Can you work these out from the model? Positions are in its coordinate system, mm. Face numbers are marked on the shaded views. Give positions to 0.01 mm unless a question says otherwise; leave off trailing zeros. Order: outer loops, then holes, each group sorted by start corner. A loop starts at its lowest first (then second) coordinate and runs counter-clockwise, first axis right, second up. Notation, with made-up numbers: (5, 76) - (29, 76) arc R23 cw to (29, 108) - close; hole circle Ø7 at (25.5, 36). An arc over 180 degrees is marked (long way). One line per question, with ' | ' between items.
```python
from build123d import *

# Parameters (mm, degrees)
F0_R        = 2.5
F1_DEPTH    = 5
F2_R        = 0.1
F3_T1_DEPTH = 5.0886751346


# Not quite as in the source:
# - a fillet or chamfer that OpenCascade refuses, or shapes differently, is made with other operations: its cross-section is extruded or revolved along the edge and cut away or added


with BuildPart() as f1:
    # F0 (on Top) → F1 (new body)
    with BuildSketch(Plane.XY):
        Polygon((2.8867513459, 5), (-2.8867513459, 5), (-5.7735026919, 0), (-2.8867513459, -5), (2.8867513459, -5), (5.7735026919, 0), align=None)
        Circle(F0_R, mode=Mode.SUBTRACT)
    extrude(amount=F1_DEPTH)

    # F2
    f2_edges = [f1.edges().sort_by_distance(p)[0] for p in [
        (4.330127, 2.5, 0),
        (0, 5, 0),
        (-4.330127, 2.5, 0),
        (-4.330127, -2.5, 0),
        (0, -5, 0),
        (4.330127, -2.5, 0),
        (-2.5, 0, 0),
        (4.330127, 2.5, 5),
        (0, 5, 5),
        (-4.330127, 2.5, 5),
        (-4.330127, -2.5, 5),
        (0, -5, 5),
        (4.330127, -2.5, 5),
        (-2.5, 0, 5),
    ]]
    fillet(f2_edges, radius=F2_R)

    # F3: fillet of radius 0.1 on 18 edges, made by hand

    # F3_s2 → F3_t1 (cut)
    with BuildSketch(Plane.XY.offset(-0.0443375673)):
        with BuildLine():
            ThreePointArc((-2.829016319, 5), (-2.879016319, 4.9866025404), (-2.9156188594, 4.95))
            Line((-2.9156188594, 4.95), (-2.8867513459, 5))
            Line((-2.8867513459, 5), (-2.829016319, 5))
        make_face()
        with BuildLine():
            ThreePointArc((-5.7446351784, 0.05), (-5.7580326381, 0), (-5.7446351784, -0.05))
            Line((-5.7446351784, -0.05), (-5.7735026919, 0))
            Line((-5.7735026919, 0), (-5.7446351784, 0.05))
        make_face()
        with BuildLine():
            ThreePointArc((2.9156188594, 4.95), (2.879016319, 4.9866025404), (2.829016319, 5))
            Line((2.829016319, 5), (2.8867513459, 5))
            Line((2.8867513459, 5), (2.9156188594, 4.95))
        make_face()
        with BuildLine():
            ThreePointArc((5.7446351784, 0.05), (5.7580326381, 0), (5.7446351784, -0.05))
            Line((5.7446351784, -0.05), (5.7735026919, 0))
            Line((5.7735026919, 0), (5.7446351784, 0.05))
        make_face()
        with BuildLine():
            ThreePointArc((-2.829016319, -5), (-2.879016319, -4.9866025404), (-2.9156188594, -4.95))
            Line((-2.9156188594, -4.95), (-2.8867513459, -5))
            Line((-2.8867513459, -5), (-2.829016319, -5))
        make_face()
        with BuildLine():
            ThreePointArc((2.9156188594, -4.95), (2.879016319, -4.9866025404), (2.829016319, -5))
            Line((2.829016319, -5), (2.8867513459, -5))
            Line((2.8867513459, -5), (2.9156188594, -4.95))
        make_face()
    extrude(amount=F3_T1_DEPTH, mode=Mode.SUBTRACT)


solid = f1.part
```
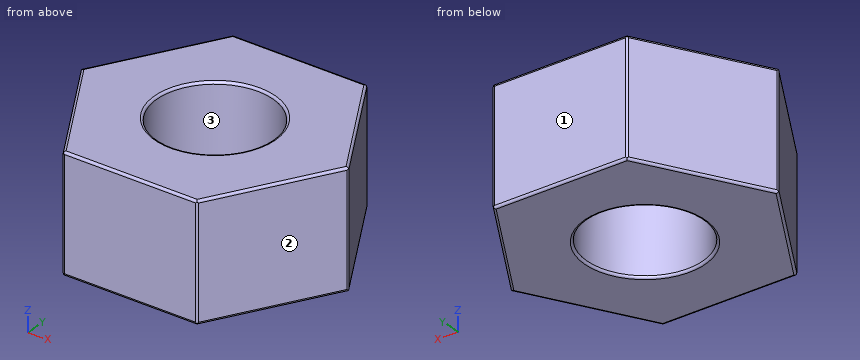
(1) Imagine slicing it at A-A (z = 1.1). List the corners of the cut face in (x, y) for me, and give its area (3 significant figures).
Answer below:
outline: (-5.74, -0.05) - (-2.92, -4.95) arc R0.1 ccw to (-2.83, -5) - (2.83, -5) arc R0.1 ccw to (2.92, -4.95) - (5.74, -0.05) arc R0.1 ccw to (5.74, 0.05) - (2.92, 4.95) arc R0.1 ccw to (2.83, 5) - (-2.83, 5) arc R0.1 ccw to (-2.92, 4.95) - (-5.74, 0.05) arc R0.1 ccw to start; hole circle Ø5 at (0, 0) | area: 67.0 mm^2
(2) If we mould it in two halves opening along X, with no side actions, what happens to the marked faces 1, 2 and 3? For each: released by +X, released by -X, zero draft, split by the parting line, or undercut.
Answer below:
face 1: zero draft | face 2: released by +X | face 3: undercut
(3) Will this pin go through, and if not, where does the flat tip stop? pin 1 (4 mm diameter, centred on x = 0, y = 0, fed in from +Z) (3 decimals).
Answer below:
pin 1: through
(4) Imagine slicing it at B-B (x = 0). List the corners of the cut face in (y, z) for me, and give its area (3 significant figures).
Answer below:
outline: (-5, 0.1) arc R0.1 ccw to (-4.9, 0) - (-2.6, 0) arc R0.1 ccw to (-2.5, 0.1) - (-2.5, 4.9) arc R0.1 ccw to (-2.6, 5) - (-4.9, 5) arc R0.1 ccw to (-5, 4.9) - close; (2.5, 0.1) arc R0.1 ccw to (2.6, 0) - (4.9, 0) arc R0.1 ccw to (5, 0.1) - (5, 4.9) arc R0.1 ccw to (4.9, 5) - (2.6, 5) arc R0.1 ccw to (2.5, 4.9) - close | area: 25.0 mm^2
(5) If I drill on line 1 (Y direction, x = 0, z = 3.85); line 2 (X direction, y = 1.5, z = 1.1); line 3 (Y direction, x = 1.5, z = 1.4), over which ranges is the centre line in solid material (lowest first)?
Answer below:
line 1: -5 to -2.5, 2.5 to 5 | line 2: -4.91 to -2, 2 to 4.91 | line 3: -5 to -2, 2 to 5
